Could you check a few things on this model? Use its own coordinates, in mm. Coordinates: 2 decimals unless noted, no trailing zeros. Write each loop counter-clockwise with the first axis right and the second up, starting at its lowest first coordinate (ties: lowest second). Pieces come first, ordered by that corner, then holes.
Item 1: I want a section at A-A on z = -17.5. Please give me the cut outline in (x, y).
Item 2: I want a section at B-B on x = -7.5. Please give me the cut outline in (y, z), then the cut area to 3 significant figures.
Item 3: If I drill on probe 1 along Z at (x, y) = (42.5, 3); probe 2 along X at (y, z) = (5.5, -17.5); probe 3 along X at (y, z) = (3.5, -16), over which ranges is the centre line in solid material (lowest first)?
Item 4: For P1, Ø4, axis at x = -42.5, z = 17.5, coming from the -Y side (1 decimal), with a flat end and sliding along its axis, tell me the tip position at first contact or that it passes through.
Item 5: I want a section at D-D on x = 43. Please give me the cut outline in (y, z), then the cut area to 3 significant figures.
Item 6: I want a section at C-C on y = 5.5. State how many separate pieces and enclosed holes the cut face has, then the cut area to 3 significant figures.
from build123d import *

# Parameters (mm, degrees)
SKETCH1_W           = 100
SKETCH1_H           = 50
SKETCH1_R           = 2.5
BOSS_EXTRUDE1_DEPTH = 10
SKETCH3_R           = 2.5
CUT_EXTRUDE1_DEPTH  = 10


with BuildPart() as part:
    # Sketch1 → Boss-Extrude1 (new body)
    with BuildSketch(Plane(origin=(0, 0, 0), x_dir=(1, 0, 0), z_dir=(0, 1, 0))):
        Rectangle(SKETCH1_W, SKETCH1_H)
        with Locations((-42.5, 17.5)):
            Circle(SKETCH1_R, mode=Mode.SUBTRACT)
        with Locations((42.5, 17.5)):
            Circle(SKETCH1_R, mode=Mode.SUBTRACT)
        with Locations((42.5, -17.5)):
            Circle(SKETCH1_R, mode=Mode.SUBTRACT)
        with Locations((-42.5, -17.5)):
            Circle(SKETCH1_R, mode=Mode.SUBTRACT)
    extrude(amount=BOSS_EXTRUDE1_DEPTH)

    # Sketch3 → Cut-Extrude1 (cut)
    with BuildSketch(Plane(origin=(0, 10, 0), x_dir=(1, 0, 0), z_dir=(0, 1, 0))):
        with Locations((-7.5, 17.5)):
            Circle(SKETCH3_R)
        with Locations((7.5, 17.5)):
            Circle(SKETCH3_R)
        with Locations((7.5, -17.5)):
            Circle(SKETCH3_R)
        with Locations((-7.5, -17.5)):
            Circle(SKETCH3_R)
    extrude(amount=-CUT_EXTRUDE1_DEPTH, mode=Mode.SUBTRACT)


solid = part.part
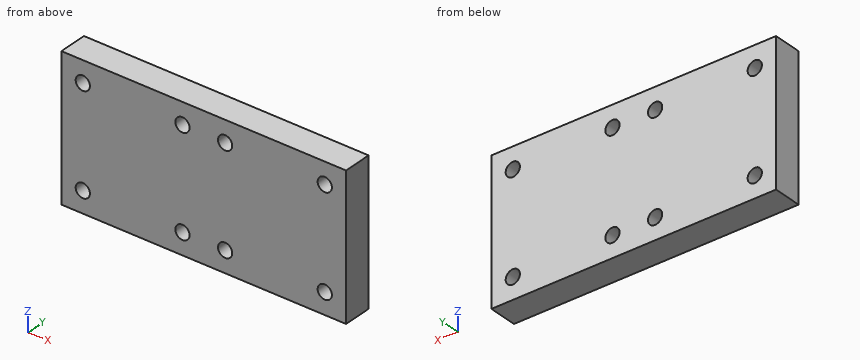
Response values:
1. outline: (-50, 0) - (-45, 0) - (-45, 10) - (-50, 10) - close; (-40, 0) - (-10, 0) - (-10, 10) - (-40, 10) - close; (-5, 0) - (5, 0) - (5, 10) - (-5, 10) - close; (10, 0) - (40, 0) - (40, 10) - (10, 10) - close; (45, 0) - (50, 0) - (50, 10) - (45, 10) - close
2. outline: (0, -25) - (10, -25) - (10, -20) - (0, -20) - close; (0, -15) - (10, -15) - (10, 15) - (0, 15) - close; (0, 20) - (10, 20) - (10, 25) - (0, 25) - close
2. area: 400 mm2
3. probe 1: z = -25 to -20, -15 to 15, 20 to 25
3. probe 2: x = -50 to -45, -40 to -10, -5 to 5, 10 to 40, 45 to 50
3. probe 3: x = -50 to -44.5, -40.5 to -9.5, -5.5 to 5.5, 9.5 to 40.5, 44.5 to 50
4. P1: passes through
5. outline: (0, -25) - (10, -25) - (10, -19.95) - (0, -19.95) - close; (0, -15.05) - (10, -15.05) - (10, 15.05) - (0, 15.05) - close; (0, 19.95) - (10, 19.95) - (10, 25) - (0, 25) - close
5. area: 402 mm2
6. separate pieces: 1
6. enclosed holes: 8
6. area: 4,840 mm2
